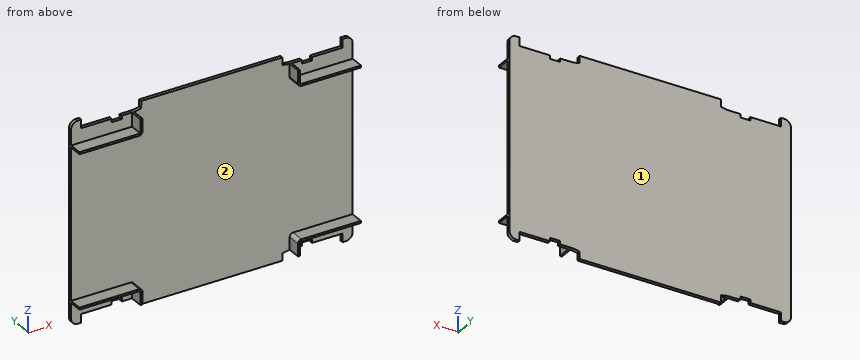
```python
from build123d import *

# Parameters (mm, degrees)
CROQUIS1_W               = 416
CROQUIS1_H               = 294
SALIENTE_EXTRUIR1_DEPTH  = 5
CORTAR_EXTRUIR1_DEPTH    = 255.750858684
REDONDEO1_R              = 10
SALIENTE_EXTRUIR3_DEPTH  = 20
REDONDEO2_R              = 5
REDONDEO2_OF_SIMETR_A3_R = 5
SIMETR_A4_DEPTH          = 5
SIMETR_A4_START          = -20
SIMETR_A4_2_DEPTH        = 20
ESCALA1_SCALE            = 2


# Read off the part's stored shape, not the designer's step: Simetría4
with BuildPart() as part:
    # Croquis1 → Saliente-Extruir1 (new body)
    with BuildSketch(Plane(origin=(0, 0, 0), x_dir=(1, 0, 0), z_dir=(0, 1, 0))):
        Rectangle(CROQUIS1_W, CROQUIS1_H)
    extrude(amount=SALIENTE_EXTRUIR1_DEPTH)

    # Croquis3 → Cortar-Extruir1 (cut, through all)
    with BuildSketch(Plane(origin=(0, 5, 0), x_dir=(1, 0, 0), z_dir=(0, 1, 0))):
        with BuildLine():
            Line((-193, 154.47), (-193, 134.47))
            Line((-193, 134.47), (-148, 134.47))
            Line((-148, 134.47), (-148, 129.47))
            Line((-148, 129.47), (-133, 129.47))
            Line((-133, 129.47), (-133, 134.47))
            Line((-133, 134.47), (-118, 134.47))
            ThreePointArc((-118, 134.47), (-111.127739024, 134.944531511), (-104.385922224, 136.359118837))
            Line((-104.385922224, 136.359118837), (-104, 156.355395091))
            Line((-104, 156.355395091), (-193, 156.355395091))
            Line((-193, 156.355395091), (-193, 154.47))
        make_face()
    cortar_extruir1 = extrude(amount=-CORTAR_EXTRUIR1_DEPTH, mode=Mode.SUBTRACT)

    # Simetría1: Cortar-Extruir1 across plane
    add(cortar_extruir1.mirror(Plane.XY), mode=Mode.SUBTRACT)

    # Redondeo1
    redondeo1_edges = [part.edges().sort_by_distance(p)[0] for p in [
        (-208, 2.5, -147),
        (208, 2.5, -147),
        (208, 2.5, 147),
        (-208, 2.5, 147),
    ]]
    fillet(redondeo1_edges, radius=REDONDEO1_R)

    # Croquis5 → Saliente-Extruir3 (add)
    with BuildSketch(Plane.XZ):
        Polygon((-208, 110.96), (-115, 110.96), (-115, 134.560081146), (-118, 134.47), (-118, 113.96), (-208, 113.96), align=None)
    saliente_extruir3 = extrude(amount=SALIENTE_EXTRUIR3_DEPTH)

    # Redondeo2
    redondeo2_edges = [part.edges().sort_by_distance(p)[0] for p in [
        (-115, -10, 110.96),
    ]]
    fillet(redondeo2_edges, radius=REDONDEO2_R)

    # Simetría3: Saliente-Extruir3 across plane
    add(saliente_extruir3.mirror(Plane.XY))

    # Redondeo2 of Simetría3
    redondeo2_of_simetr_a3_edges = [part.edges().sort_by_distance(p)[0] for p in [
        (-115, -10, -110.96),
    ]]
    fillet(redondeo2_of_simetr_a3_edges, radius=REDONDEO2_OF_SIMETR_A3_R)

    # Simetría4 outline → Simetría4 (cut)
    with BuildSketch(Plane(origin=(0, 0, 0), x_dir=(1, 0, 0), z_dir=(0, 1, 0))):
        with BuildLine():
            Line((148, 134.47), (193, 134.47))
            Line((193, 134.47), (193, 147))
            Line((193, 147), (104.180556361, 147))
            Line((104.180556361, 147), (104.385922224, 136.359118837))
            ThreePointArc((104.385922224, 136.359118837), (111.127739024, 134.944531511), (118, 134.47))
            Line((118, 134.47), (133, 134.47))
            Line((133, 134.47), (133, 129.47))
            Line((133, 129.47), (148, 129.47))
            Line((148, 129.47), (148, 134.47))
        make_face()
        with BuildLine():
            Line((133, -134.47), (118, -134.47))
            ThreePointArc((118, -134.47), (111.127739024, -134.944531511), (104.385922224, -136.359118837))
            Line((104.385922224, -136.359118837), (104.180556361, -147))
            Line((104.180556361, -147), (193, -147))
            Line((193, -147), (193, -134.47))
            Line((193, -134.47), (148, -134.47))
            Line((148, -134.47), (148, -129.47))
            Line((148, -129.47), (133, -129.47))
            Line((133, -129.47), (133, -134.47))
        make_face()
    extrude(amount=SIMETR_A4_DEPTH, mode=Mode.SUBTRACT)

    # Simetr_a4 2 outline → Simetr_a4 2 (add)
    with BuildSketch(Plane(origin=(0, 0, 0), x_dir=(1, 0, 0), z_dir=(0, 1, 0)).offset(SIMETR_A4_START)):
        with BuildLine():
            Line((208, -113.96), (208, -110.96))
            Line((208, -110.96), (120, -110.96))
            ThreePointArc((120, -110.96), (116.464466094, -112.424466094), (115, -115.96))
            Line((115, -115.96), (115, -134.560081146))
            Line((115, -134.560081146), (118, -134.47))
            Line((118, -134.47), (118, -113.96))
            Line((118, -113.96), (208, -113.96))
        make_face()
        with BuildLine():
            ThreePointArc((118, 134.47), (116.499323935, 134.492525361), (115, 134.560081146))
            Line((115, 134.560081146), (115, 115.96))
            ThreePointArc((115, 115.96), (116.464466094, 112.424466094), (120, 110.96))
            Line((120, 110.96), (208, 110.96))
            Line((208, 110.96), (208, 113.96))
            Line((208, 113.96), (118, 113.96))
            Line((118, 113.96), (118, 134.47))
        make_face()
    extrude(amount=SIMETR_A4_2_DEPTH)


with BuildPart() as part_1:
    # Escala1: scaled about (-0.000170943, 1.954243012, 0.000197364)
    add(part.part.scale(ESCALA1_SCALE).moved(Location((0.000170943, -1.954243012, -0.000197364))))


solid = part_1.part
```
The listing builds one solid part. Answer for the finished solid, in the listing's coordinates (mm). Face numbers are marked on the shaded views. A direction names the side the tool comes from. Give positions to 0.01 mm unless a question says otherwise; leave off trailing zeros. Order: outer loops, then holes, each group sorted by start corner. A loop starts at its lowest first (then second) coordinate and runs counter-clockwise, first axis right, second up.
1) For the marked faces 1 and 2, determine the directions among +Z, -Z, +X, -X, +Y, -Y from which every point of the face is accessible in a straight line to the end or side of a thin tool.
Reported:
face 1: +Z, -Z, +X, -X, +Y
face 2: -Y
2) Find section B-B on z = 243. Write down the section's boundary in (x, y).
Reported:
outline: (-416, -1.95) - (-236, -1.95) - (-236, -41.95) - (-230, -41.95) - (-230, -1.95) - (230, -1.95) - (230, -41.95) - (236, -41.95) - (236, -1.95) - (416, -1.95) - (416, 8.05) - (-416, 8.05) - close
3) Find section C-C on x = 307. Write down the section's boundary in (y, z), then the cut area to 3 significant figures.
Reported:
outline: (-41.95, -227.92) - (-1.95, -227.92) - (-1.95, -268.94) - (8.05, -268.94) - (8.05, 268.94) - (-1.95, 268.94) - (-1.95, 227.92) - (-41.95, 227.92) - (-41.95, 221.92) - (-1.95, 221.92) - (-1.95, -221.92) - (-41.95, -221.92) - close
area: 5,860 mm2
4) Consider line 1 along Z through (x, y) = (-263, -39); line 2 along Y through (x, z) = (-242.5, -186); line 3 along Z through (x, y) = (-234.5, -28). Determine where each line is inside the solid, lowest interval first.
Reported:
line 1: z = -227.92 to -221.92, 221.92 to 227.92
line 2: y = -1.95 to 8.05
line 3: z = -268.99 to -223.57, 223.57 to 268.98
5) Given P1, Ø12, axis at y = -20, z = 251.5, coming from the -X side; P2, Ø12, axis at x = -355, y = -15, coming from the +Z side; P3, Ø18.5, axis at y = -16.5, z = 244, coming from the +X side, each flat-ended and moving along its own axis, determine where each tip first touches the part or whether it passes through.
Reported:
P1: stops at x = -236
P2: stops at z = 227.92
P3: stops at x = 236
6) Find section D-D on x = 91.5. Write down the section's boundary in (y, z).
Reported:
outline: (-1.95, -294) - (8.05, -294) - (8.05, 294) - (-1.95, 294) - close
7) Find section A-A on y = -32. Write down the section's boundary in (x, z).
Reported:
outline: (-416, -227.92) - (-236, -227.92) - (-236, -268.94) - (-230, -269.12) - (-230, -231.92) arc R10 ccw to (-240, -221.92) - (-416, -221.92) - close; (-416, 221.92) - (-240, 221.92) arc R10 ccw to (-230, 231.92) - (-230, 269.12) - (-236, 268.94) - (-236, 227.92) - (-416, 227.92) - close; (230, -269.12) arc R100 cw to (236, -268.94) - (236, -227.92) - (416, -227.92) - (416, -221.92) - (240, -221.92) arc R10 ccw to (230, -231.92) - close; (230, 231.92) arc R10 ccw to (240, 221.92) - (416, 221.92) - (416, 227.92) - (236, 227.92) - (236, 268.94) - (230, 269.12) - close
